```python
from build123d import *

# Parameters (mm, degrees)
SKETCH_1_R          = 1.5
EXTRUDE_1_DEPTH     = 14
SKETCH_2_R          = 10
SKETCH_2_R_2        = 8
EXTRUDE_2_DEPTH     = 20
CUT_EXTRUDE_4_DEPTH = 20
SKETCH_6_R          = 1.5
CUT_EXTRUDE_5_DEPTH = 10


with BuildPart() as part:
    # 草图1 → 凸台-拉伸1 (new body)
    with BuildSketch(Plane(origin=(0, 0, 0), x_dir=(1, 0, 0), z_dir=(0, 1, 0))):
        with BuildLine():
            Line((0, 0), (19, 0))
            Line((19, 0), (19, 64))
            ThreePointArc((19, 64), (0, 66.760766922), (-19, 64))
            Line((-19, 64), (-19, 0))
            Line((-19, 0), (0, 0))
        make_face()
        with Locations(Location((-16.171572875, 61.171572875, 0), (0, 0, 270))):
            Circle(SKETCH_1_R, mode=Mode.SUBTRACT)
        with Locations(Location((16.171572875, 61.171572875, 0), (0, 0, 270))):
            Circle(SKETCH_1_R, mode=Mode.SUBTRACT)
        with Locations(Location((-16.171572875, 2.828427125, 0), (0, 0, 270))):
            Circle(SKETCH_1_R, mode=Mode.SUBTRACT)
        with Locations(Location((16.171572875, 2.828427125, 0), (0, 0, 270))):
            Circle(SKETCH_1_R, mode=Mode.SUBTRACT)
        with BuildLine():
            Line((-16.171572875, 57.171572875), (-16.171572875, 6.828427125))
            ThreePointArc((-16.171572875, 6.828427125), (-13.343145751, 5.656854249), (-12.171572875, 2.828427125))
            Line((-12.171572875, 2.828427125), (12.171572875, 2.828427125))
            ThreePointArc((12.171572875, 2.828427125), (13.343145751, 5.656854249), (16.171572875, 6.828427125))
            Line((16.171572875, 6.828427125), (16.171572875, 57.171572875))
            ThreePointArc((16.171572875, 57.171572875), (13.0281615, 58.697918711), (12.283716556, 62.112090413))
            ThreePointArc((12.283716556, 62.112090413), (0, 63.371324523), (-12.283716556, 62.112090413))
            ThreePointArc((-12.283716556, 62.112090413), (-13.0281615, 58.697918711), (-16.171572875, 57.171572875))
        make_face(mode=Mode.SUBTRACT)
    extrude(amount=EXTRUDE_1_DEPTH)

    # 草图2 → 凸台-拉伸2 (add)
    with BuildSketch(Plane.XY):
        with Locations(Location((0, 7, 0), (0, 0, 135.572995999))):
            Circle(SKETCH_2_R)
        with Locations(Location((0, 7, 0), (0, 0, 241.044975628))):
            Circle(SKETCH_2_R_2, mode=Mode.SUBTRACT)
    extrude(amount=EXTRUDE_2_DEPTH)

    # 草图3 → 切除-拉伸4 (cut, symmetric)
    with BuildSketch(Plane(origin=(0, 0, 0), x_dir=(1, 0, 0), z_dir=(0, 1, 0))):
        Polygon((0, -1.124822793), (7, -5.124822793), (7, -8.124822793), (0, -4.124822793), (-7, -8.124822793), (-7, -5.124822793), align=None)
        Polygon((0, -12.124822793), (7, -16.124822793), (7, -19.124822793), (0, -15.124822793), (-7, -19.124822793), (-7, -16.124822793), align=None)
    extrude(amount=CUT_EXTRUDE_4_DEPTH, both=True, mode=Mode.SUBTRACT)

    # 草图6 → 切除-拉伸5 (cut)
    with BuildSketch(Plane(origin=(0, 0, 0), x_dir=(1, 0, 0), z_dir=(0, 1, 0))):
        with Locations(Location((0, -10, 0), (0, 0, 270))):
            Circle(SKETCH_6_R)
    extrude(amount=-CUT_EXTRUDE_5_DEPTH, mode=Mode.SUBTRACT)


solid = part.part
```
Build history of the part. All positions in model axes, mm. A direction names the side the tool comes from. Round coordinates to 2 decimals unless told otherwise and drop trailing zeros. Write each loop counter-clockwise with the first axis right and the second up, starting at its lowest first coordinate (ties: lowest second). Pieces come first, ordered by that corner, then holes. Notation, with made-up numbers: (-34, 87) -> (-5, 87) arc R19 ccw to (-5, 117) -> close; hole circle Ø5 at (-25, 42). An arc over 180 degrees is marked (long way). Put each result on its own line as item: value.
Item 1: Two-plate mould, pull along Z, no slides. Class faces 4 (the face through (7, 12, 7)), 5 (the face through (0, -2, 0)), 6 (the face through (-17, 14, -36)): pulls with the +Z half, pulls with the -Z half, needs draft (parallel to the pull), parting line crosses it, or undercut.
Here are the results:
face 4: undercut
face 5: pulls with the -Z half
face 6: needs draft
Item 2: Wall check: probe 1 along Z at (x, y) = (0, -2); probe 2 along X at (y, z) = (2.5, -25.5); probe 3 along Z at (x, y) = (16.5, 11.25). Give the ranges that are in metal, low to high. Write a range as from..to.
Here are the results:
probe 1: z = 0..1.12, 4.12..8.5, 11.5..12.12, 15.12..20
probe 2: x = -19..-16.17, 16.17..19
probe 3: z = -64.69..-62.64, -59.71..-4.29, -1.36..0
Item 3: Slice it at D-D, the plane z = 10. Give the cut face in (x, y), plus the area to 3 significant figures.
Here are the results:
outline: (-1.5, -2.89) -> (-1.5, -0.86) arc R8 cw (long way) to (1.5, -0.86) -> (1.5, -2.89) arc R10 ccw (long way) to start
area: 107 mm^2
Item 4: Slice it at A-A, the plane y = 7. Give the cut face in (x, z), plus the area to 3 significant figures.
Here are the results:
outline: (-19, -64) arc R66.76 ccw to (19, -64) -> (19, 0) -> (10, 0) -> (10, 20) -> (8, 20) -> (8, 0) -> (-8, 0) -> (-8, 20) -> (-10, 20) -> (-10, 0) -> (-19, 0) -> close; hole circle Ø3 at (-16.17, -61.17); hole circle Ø3 at (-16.17, -2.83); hole (-16.17, -57.17) arc R4 cw to (-12.28, -62.11) arc R60.54 ccw to (12.28, -62.11) arc R4 cw to (16.17, -57.17) -> (16.17, -6.83) arc R4 cw to (12.17, -2.83) -> (-12.17, -2.83) arc R4 cw to (-16.17, -6.83) -> close; hole circle Ø3 at (16.17, -61.17); hole circle Ø3 at (16.17, -2.83)
area: 674 mm^2
Item 5: Slice it at C-C, the plane x = -5. Count the separate pieces of the cut face and the enclosed holes in it, plus the area to 3 significant figures.
Here are the results:
separate pieces: 6
enclosed holes: 0
area: 155 mm^2
Item 6: Flat gauge pins, fed straight in: P1, Ø2.5, axis at y = 1.5, z = 18, coming from the -X side; P2, Ø3, axis at x = -2, y = 13, coming from the -Z side; P3, Ø3.5, axis at x = -12, y = 5, coming from the +Z side; P4, Ø2, axis at x = -15, z = -49, coming from the -Y side. Where does each tip first touch, or does it go through?
Here are the results:
P1: stops at x = -9.05
P2: stops at z = -66.76
P3: stops at z = 0
P4: passes through
Item 7: Slice it at B-B, the plane z = -23. Give the cut face in (x, y).
Here are the results:
outline: (-19, 0) -> (-16.17, 0) -> (-16.17, 14) -> (-19, 14) -> close; (16.17, 0) -> (19, 0) -> (19, 14) -> (16.17, 14) -> close
Item 8: Tool access for faces 1 (the face through (0.07, -1.92, 8.5)), 2 (the face through (-3.549, -0.66, 3.153)), 3 (the face through (0, 7, 0)): list every direction of +Z, -Z, +X, -X, +Y, -Y with a clear straight run to the whole face (end or side of a thin tool).
Here are the results:
face 1: -Y
face 2: +Y, -Y
face 3: +Z
